The listing builds one solid part. Answer for the finished solid, in the listing's coordinates (mm). Face numbers are marked on the shaded views. Round coordinates to 2 decimals unless told otherwise and drop trailing zeros. Write each loop counter-clockwise with the first axis right and the second up, starting at its lowest first coordinate (ties: lowest second). Pieces come first, ordered by that corner, then holes.
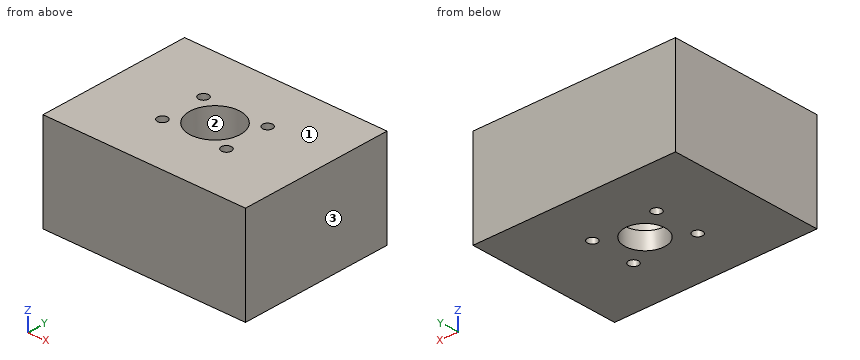
from build123d import *

# Parameters (mm, degrees)
F0_W           = 132.338822
F0_H           = 100.486502
F1_DEPTH       = 63.5
F3_D           = 26.2255
F3_CBORE_D     = 33.02
F3_CBORE_DEPTH = 52.324
F5_D           = 6.5278


with BuildPart() as f1:
    # F0 (on Top) → F1 (new body)
    with BuildSketch(Plane.XY):
        Rectangle(F0_W, F0_H)
    extrude(amount=F1_DEPTH)

    # F3 (through all)
    with Locations(Plane.XY.offset(63.5)):
        with Locations((0, 0)):
            CounterBoreHole(F3_D / 2, F3_CBORE_D / 2, F3_CBORE_DEPTH)

    # F5 (through all)
    with Locations(Plane(origin=(0, 0, 0), x_dir=(1, 0, 0), z_dir=(0, 0, -1))):
        with Locations((-20.955, 14.605), (-20.955, -14.605), (20.955, -14.605), (20.955, 14.605)):
            Hole(F5_D / 2)


solid = f1.part
1. Section B-B on y = 0 is taken. Determine the outline of the cut face in (x, z).
Geometry says:
outline: (-66.17, 0) - (-13.11, 0) - (-13.11, 11.18) - (-16.51, 11.18) - (-16.51, 63.5) - (-66.17, 63.5) - close; (13.11, 0) - (66.17, 0) - (66.17, 63.5) - (16.51, 63.5) - (16.51, 11.18) - (13.11, 11.18) - close
2. Section A-A on x = 0 is taken. Determine the outline of the cut face in (y, z).
Geometry says:
outline: (-50.24, 0) - (-13.11, 0) - (-13.11, 11.18) - (-16.51, 11.18) - (-16.51, 63.5) - (-50.24, 63.5) - close; (13.11, 0) - (50.24, 0) - (50.24, 63.5) - (16.51, 63.5) - (16.51, 11.18) - (13.11, 11.18) - close
3. Given pin 1 (10 mm diameter, centred on x = -4.5, y = -4, fed in from +Z), flat-ended and moving along its own axis, determine where the tip first touches the part or whether it passes through.
Geometry says:
pin 1: passes through
4. Section D-D on z = 17 is taken. Determine the outline of the cut face in (x, y) (3 decimals), plus the area to 3 significant figures.
Geometry says:
outline: (-66.169, -50.243) - (66.169, -50.243) - (66.169, 50.243) - (-66.169, 50.243) - close; hole circle Ø6.528 at (-20.955, -14.605); hole circle Ø6.528 at (-20.955, 14.605); hole circle Ø33.02 at (0, 0); hole circle Ø6.528 at (20.955, -14.605); hole circle Ø6.528 at (20.955, 14.605)
area: 12,300 mm2
5. For a pull along X with two mould halves and no side action, classify the marked faces 1, 2 and 3 as released by +X, released by -X, zero draft, split by the parting line, or undercut.
Geometry says:
face 1: zero draft
face 2: undercut
face 3: released by +X
6. Section C-C on x = -22 is taken. Determine the outline of the cut face in (y, z).
Geometry says:
outline: (-50.24, 0) - (-17.7, 0) - (-17.7, 63.5) - (-50.24, 63.5) - close; (-11.51, 0) - (11.51, 0) - (11.51, 63.5) - (-11.51, 63.5) - close; (17.7, 0) - (50.24, 0) - (50.24, 63.5) - (17.7, 63.5) - close
7. Straight lines are drawn through the part: line 1 along Y through (x, z) = (0, 8); line 2 along Y through (x, z) = (21, 54); line 3 along X through (y, z) = (-1, 12.5). For each, find the intervals that lie inside material, in ascending order.
Geometry says:
line 1: y = -50.24 to -13.11, 13.11 to 50.24
line 2: y = -50.24 to -17.87, -11.34 to 11.34, 17.87 to 50.24
line 3: x = -66.17 to -16.48, 16.48 to 66.17
